Read the model definition and answer for the solid it produces. Units are mm, in the model's axes. A direction names the side the tool comes from. Round coordinates to 2 decimals unless told otherwise and drop trailing zeros. Order: outer loops, then holes, each group sorted by start corner. A loop starts at its lowest first (then second) coordinate and runs counter-clockwise, first axis right, second up. Notation, with made-up numbers: (41.5, -14.75) -> (91.5, -14.75) arc R5 ccw to (91.5, -7.75) -> close; hole circle Ø6 at (11.5, 59.25). An arc over 180 degrees is marked (long way). Answer as a JSON object with one key per item and string values. Group by question number.
Item 1: Consider probe 1 along Z at (x, y) = (-42.5, 10.75) (3 decimals); probe 2 along Z at (x, y) = (-13, 10.75). Determine where each line is inside the solid, lowest interval first. Write a range as from..to.
Item 2: For faces 4 (the flat face through (40, 18, -3)), 5 (the cylindrical face through (-21.797, 13.479, 21.859)), 6 (the flat face through (50, 12, -1)), determine the directions among +Z, -Z, +X, -X, +Y, -Y from which every point of the face is accessible in a straight line to the end or side of a thin tool.
Item 3: Given P1, Ø1.5, axis at x = -2.5, z = -15, coming from the +Y side; P2, Ø6, axis at x = -13.5, z = -0.5, coming from the -Y side, each flat-ended and moving along its own axis, determine where each tip first touches the part or whether it passes through.
Item 4: Section C-C, the plane z = -42.5 is taken. Write down the section's boundary in (x, y) (3 decimals), plus the area to 3 significant figures.
Item 5: Section A-A, the plane y = 10 is taken. Write down the section's boundary in (x, z) (3 decimals), plus the area to 3 significant figures.
Item 6: Section B-B, the plane x = -42.5 is taken. Write down the section's boundary in (y, z) (3 decimals).
Item 7: Section D-D, the plane x = 17 is taken. Write down the section's boundary in (y, z) (3 decimals).
Item 8: The mould has two halves that part along Z. Classify faces 1 (the cylindrical face through (48.859, 12.296, 48.797)), 2 (the flat face through (1, 5, 1)), 3 (the flat face through (29.575, 17, 15)): pulls with the +Z half, pulls with the -Z half, needs draft (parallel to the pull), parting line crosses it, or undercut.
Autodesk Inventor part; units mm, degrees
ref_plane "Work Plane2" through (-27, 15, 23) normal (0, 0, -1) x (-1, 0, 0)
ref_plane "YZ Plane" through (0, 0, 0) normal (1, 0, 0) x (0, 1, 0)
ref_plane "XZ Plane" through (0, 0, 0) normal (0, 1, 0) x (-1, 0, 0)
sketch "peltier" plane through (0, 0, 0) normal (0, 0, 1) x (1, 0, 0)
  line L0 (7.1779, -44.0485) -> (-50.9721, -44.0485)
  line L1 (-50.9721, -44.0485) -> (-50.9721, -102.2985)
  line L2 (-50.9721, -102.2985) -> (7.1779, -102.2985)
  line L3 (7.1779, -102.2985) -> (7.1779, -44.0485)
  point P0 (-21.8971, -73.1735)
  point P1 (-21.8971, -73.1735)
  dimension "d0" = 58.25
  dimension "d1" = 58.15
sketch "Sketch1" plane through (0, 0, 0) normal (0, 1, 0) x (-1, 0, 0)
  line L0 (-46, 50) -> (46, 50)
  line L1 (50, 46) -> (50, -46)
  line L2 (46, -50) -> (-46, -50)
  line L3 (-50, -46) -> (-50, 46)
  line L4 (-50, 50) -> (50, -50) construction
  line L5 (50, 50) -> (-50, -50) construction
  line L6 (-29.575, 29.575) -> (29.575, 29.575)
  line L7 (29.575, 29.575) -> (29.575, -29.575)
  line L8 (29.575, -29.575) -> (-29.575, -29.575)
  line L9 (-29.575, -29.575) -> (-29.575, 29.575)
  line L10 (-29.575, 29.575) -> (29.575, -29.575) construction
  line L11 (29.575, 29.575) -> (-29.575, -29.575) construction
  line L12 (-29.575, 0) -> (-50, 0)
  line L13 (-19, 23) -> (19, 23)
  line L14 (23, 19) -> (23, -19)
  line L15 (19, -23) -> (-19, -23)
  line L16 (-23, -19) -> (-23, 19)
  line L17 (-23, 23) -> (23, -23) construction
  line L18 (23, 23) -> (-23, -23) construction
  arc A0 (50, 46) -> (46, 50) centre (46, 46) ccw
  arc A1 (-46, 50) -> (-50, 46) centre (-46, 46) ccw
  arc A2 (-50, -46) -> (-46, -50) centre (-46, -46) ccw
  arc A3 (46, -50) -> (50, -46) centre (46, -46) ccw
  arc A4 (23, 19) -> (19, 23) centre (19, 19) ccw
  arc A5 (-19, 23) -> (-23, 19) centre (-19, 19) ccw
  arc A6 (-23, -19) -> (-19, -23) centre (-19, -19) ccw
  arc A7 (19, -23) -> (23, -19) centre (19, -19) ccw
  line L19 (-29.575, 0) -> (-29.575, -3)
  line L20 (-29.575, -3) -> (-50, -3)
  line L21 (-50, -3) -> (-50, 3)
  line L22 (-50, 3) -> (-29.575, 3)
  line L23 (-29.575, 3) -> (-29.575, -3)
  circle A8 centre (13, 0) radius 6.35
  circle A9 centre (-13, 0) radius 6.35
  line L24 (29.075, 29.125) -> (-29.075, 29.125)
  line L25 (-29.075, 29.125) -> (-29.075, -29.125)
  line L26 (-29.075, -29.125) -> (29.075, -29.125)
  line L27 (29.075, -29.125) -> (29.075, 29.125)
  point P0 (0, 0)
  point P1 (0, 0)
  dimension "d2" = 100
  dimension "d3" = 100
  dimension "d4" = 0.5
  dimension "d5" = 4
  dimension "d6" = 46
  dimension "d7" = 46
  dimension "d8" = 4
  dimension "d13" = 3
  dimension "d14" = 6
  dimension "d17" = 12.7
  dimension "d18" = 13
  dimension "d19" = 13
  dimension "d20" = 12.7
extrude "Extrusion1" add sketch "Sketch1" along normal blind 20 contours L0 A0 L1 A3 L2 A2 L3 L20 L9 L8 L7 L6 L22 A1
extrude "Extrusion2" add sketch "Sketch1" along normal blind 15 contours L22 L9 L12 L3 | L12 L9 L20 L3 | L9 L6 L7 L8 | L27 L26 L25 L24
extrude "Extrusion3" add sketch "Sketch1" along normal blind 12 contours L13 A4 L14 A7 L15 A6 L16 A5
sketch "Sketch2" plane through (0, 15, 0) normal (0, 1, 0) x (1, 0, 0)
  line L0 (-29.575, -29.575) -> (-29.575, 29.575)
  line L1 (29.575, -29.575) -> (-29.575, -29.575)
  line L2 (29.575, -3) -> (29.575, -29.575)
  line L3 (50, -3) -> (29.575, -3)
  line L4 (50, -3) -> (50, 3)
  line L5 (29.575, 3) -> (50, 3)
  line L6 (29.575, 29.575) -> (29.575, 3)
  line L7 (-29.575, 29.575) -> (29.575, 29.575)
  line L8 (23, 19) -> (23, -19)
  arc A0 (19, -23) -> (23, -19) centre (19, -19) ccw
  line L9 (19, -23) -> (-19, -23)
  arc A1 (-23, -19) -> (-19, -23) centre (-19, -19) ccw
  line L10 (-23, -19) -> (-23, 19)
  arc A2 (-19, 23) -> (-23, 19) centre (-19, 19) ccw
  line L11 (-19, 23) -> (19, 23)
  arc A3 (23, 19) -> (19, 23) centre (19, 19) ccw
  line L12 (23, -27) -> (-23, -27)
  line L13 (-27, -23) -> (-27, 23)
  line L14 (-23, 27) -> (23, 27)
  line L15 (27, 23) -> (27, -23)
  line L16 (27, -27) -> (-27, 27) construction
  line L17 (-27, -27) -> (27, 27) construction
  arc A4 (-27, -23) -> (-23, -27) centre (-23, -23) ccw
  arc A5 (-23, 27) -> (-27, 23) centre (-23, 23) ccw
  arc A6 (27, 23) -> (23, 27) centre (23, 23) ccw
  arc A7 (23, -27) -> (27, -23) centre (23, -23) ccw
  point P0 (0, 0)
  dimension "d21" = 4
  dimension "d25" = 4
  dimension "d29" = 4
ref_plane "Work Plane2" through (-27, 15, 23) normal (0, 0, -1) x (-1, 0, 0)
sketch "Sketch4" plane through (-27, 15, 23) normal (0, 0, -1) x (-1, 0, 0)
  circle A0 centre (0, 0) radius 1
  point P0 (-27, -15)
  dimension "d26" = 2
sweep "Sweep2" cut profiles "Sketch4" path "Sketch2" path curves L13 A5 L14 A6 L15 A7 L12 A4
thread "Thread1"
thread "Thread2"
move faces "Move1" translate (0, 5, 0) faces at (-3.5828, 0, -35.3125)
move faces "Move2" translate (0, -0.2, 0) faces at (-43.1917, 20, 9.8583)
fillet "Fillet1" radius 2 2 edges at (39.7875, 15, 3) (39.7875, 15, -3)
sketch "Sketch6" plane through (-46, 19.8, -50) normal (0, 1, 0) x (1, 0, 0)
  line L0 (96, -96) -> (96, -53)
  line L1 (96, -53) -> (75.575, -53)
  line L2 (75.575, -53) -> (75.575, -79.575)
  line L3 (75.575, -79.575) -> (16.425, -79.575)
  line L4 (16.425, -79.575) -> (16.425, -20.425)
  line L5 (16.425, -20.425) -> (75.575, -20.425)
  line L6 (75.575, -20.425) -> (75.575, -47)
  line L7 (75.575, -47) -> (96, -47)
  line L8 (96, -47) -> (96, -4)
  arc A0 (96, -4) -> (92, 0) centre (92, -4) ccw
  line L9 (92, 0) -> (0, 0)
  arc A1 (0, 0) -> (-4, -4) centre (0, -4) ccw
  line L10 (-4, -4) -> (-4, -96)
  arc A2 (-4, -96) -> (0, -100) centre (0, -96) ccw
  line L11 (0, -100) -> (92, -100)
  arc A3 (92, -100) -> (96, -96) centre (92, -96) ccw
  line L12 (3.5, -92.5) -> (88.5, -92.5)
  line L13 (88.5, -92.5) -> (88.5, -7.5)
  line L14 (88.5, -7.5) -> (3.5, -7.5)
  line L15 (3.5, -7.5) -> (3.5, -92.5)
  line L16 (3.5, -92.5) -> (88.5, -7.5) construction
  line L17 (88.5, -92.5) -> (3.5, -7.5) construction
  circle A4 centre (3.5, -92.5) radius 3.175
  circle A5 centre (3.5, -7.5) radius 3.175
  circle A6 centre (88.5, -92.5) radius 3.175
  circle A7 centre (88.5, -7.5) radius 3.175
  point P0 (46, -50)
  dimension "d43" = 6.35
  dimension "d45" = 85
  dimension "d46" = 85
  dimension "d49" = 85
  dimension "d52" = 85
extrude "Extrusion4" cut sketch "Sketch6" against normal up to surface (14.8 mm away) contours A6 L12 L13 | L13 L12 A6 | A7 L14 L13 | L13 L14 A7 | A4 L15 L12 | L12 L15 A4 | A5 L15 L14 | L14 L15 A5
properties part number "inf_soporte"
Values found:
{
 "1": {"probe 1": "-50..-45.675, -39.325..39.325, 45.675..50", "probe 2": "-50..-6.35, 6.35..50"},
 "2": {"face 4": "+X, +Y", "face 5": "+Y", "face 6": "+Z, -Z, +X, +Y, -Y"},
 "3": {"P1": "y = 12", "P2": "through"},
 "4": {"outline": "(-50, 5) -> (-45.675, 5) -> (-45.675, 19.8) -> (-50, 19.8) -> close; (-39.325, 5) -> (39.325, 5) -> (39.325, 19.8) -> (-39.325, 19.8) -> close; (45.675, 5) -> (50, 5) -> (50, 19.8) -> (45.675, 19.8) -> close", "area": "1,290 mm2"},
 "5": {"outline": "(-50, -46) arc R4 ccw to (-46, -50) -> (46, -50) arc R4 ccw to (50, -46) -> (50, 46) arc R4 ccw to (46, 50) -> (-46, 50) arc R4 ccw to (-50, 46) -> close; hole circle Ø6.35 at (-42.5, -42.5); hole circle Ø6.35 at (-42.5, 42.5); hole circle Ø12.7 at (-13, 0); hole circle Ø12.7 at (13, 0); hole circle Ø6.35 at (42.5, -42.5); hole circle Ø6.35 at (42.5, 42.5)", "area": "9,610 mm2"},
 "6": {"outline": "(5, -50) -> (19.8, -50) -> (19.8, -45.675) -> (5, -45.675) -> close; (5, -39.325) -> (19.8, -39.325) -> (19.8, 39.325) -> (5, 39.325) -> close; (5, 45.675) -> (19.8, 45.675) -> (19.8, 50) -> (5, 50) -> close"},
 "7": {"outline": "(5, -50) -> (19.8, -50) -> (19.8, -29.575) -> (15, -29.575) -> (15, -28) arc R1 cw to (15, -26) -> (15, -23) -> (12, -23) -> (12, -4.932) -> (5, -4.932) -> close; (5, 4.932) -> (12, 4.932) -> (12, 23) -> (15, 23) -> (15, 26) arc R1 cw to (15, 28) -> (15, 29.575) -> (19.8, 29.575) -> (19.8, 50) -> (5, 50) -> close"},
 "8": {"face 1": "pulls with the +Z half", "face 2": "needs draft", "face 3": "undercut"}
}
